Read the model definition and answer for the solid it produces. Units are mm, in the model's axes. A direction names the side the tool comes from. Give positions to 0.01 mm unless a question says otherwise; leave off trailing zeros. Order: outer loops, then holes, each group sorted by start corner. A loop starts at its lowest first (then second) coordinate and runs counter-clockwise, first axis right, second up. Notation, with made-up numbers: (16.25, -10.5) - (26.25, -10.5) arc R20 cw to (26.25, 1.5) - close; hole circle Ø6 at (7.25, 62.25). An arc over 180 degrees is marked (long way). Return JSON: item names as keys, results as strings.
```python
from build123d import *

# Parameters (mm, degrees)
SKETCH_3_R          = 1.25
CUT_EXTRUDE_1_DEPTH = 15.361406616
CHAMFER_1_SIZE      = 0.2


with BuildPart() as part:
    # 草图2 → 旋转1 (revolve)
    with BuildSketch(Plane.XY, mode=Mode.PRIVATE) as revolve_1_sk:
        Polygon((0, 3), (0, 4.5), (2, 4.5), (2, 10), (4.5, 10), (4.5, 1.5), (3.5, 1.5), (3.5, 3), align=None)
    revolve(revolve_1_sk.sketch.rotate(Axis((0, 0, 0), (1, 0, 0)), 90), axis=Axis((0, 0, 0), (1, 0, 0)))

    # 草图3 → 切除-拉伸1 (cut, through all)
    with BuildSketch(Plane.ZY.offset(-2)):
        with Locations((4.949747468, 4.949747468)):
            Circle(SKETCH_3_R)
        with Locations((4.949747468, -4.949747468)):
            Circle(SKETCH_3_R)
        with Locations((-4.949747468, -4.949747468)):
            Circle(SKETCH_3_R)
        with Locations((-4.949747468, 4.949747468)):
            Circle(SKETCH_3_R)
    extrude(amount=-CUT_EXTRUDE_1_DEPTH, mode=Mode.SUBTRACT)

    # 倒角1
    chamfer_1_edges = [part.edges().sort_by_distance(p)[0] for p in [
        (4.5, 0, -1.5),
        (4.5, 0, -10),
        (2, 0, -10),
        (0, 0, -4.5),
    ]]
    chamfer(chamfer_1_edges, length=CHAMFER_1_SIZE)


solid = part.part
```
Q1. A cutting plane is placed at C-C (x = 1). Write down the section's boundary in (y, z).
Values:
{"outline": "circle Ø9 at (0, 0); hole circle Ø6 at (0, 0)"}
Q2. For faces 4 (the cylindrical face through (1.11, -3.04, -3.32)), 5 (the flat face through (0, 1, 3)), determine the directions among +Z, -Z, +X, -X, +Y, -Y from which every point of the face is accessible in a straight line to the end or side of a thin tool.
Values:
{"face 4": "-X", "face 5": "+Z, -Z, -X, +Y, -Y"}
Q3. A cutting plane is placed at D-D (y = 4). Give the number of separate pieces and of enclosed holes in the cut face, and give its area (3 significant figures).
Values:
{"separate pieces": "3", "enclosed holes": "0", "area": "45.8 mm²"}
Q4. Consider L1, parallel to X at y = 2.25, z = 1; L2, parallel to Z at x = 1.9, y = 1.5; L3, parallel to Y at x = 3.1, z = 5.5. Determine where each line is inside the solid, lowest interval first.
Values:
{"L1": "x = 3.5 to 4.5", "L2": "z = -4.24 to -2.6, 2.6 to 4.24", "L3": "y = -8.35 to -6.07, -3.83 to 3.83, 6.07 to 8.35"}
Q5. Determine the mould class of faces 1 (the flat face through (4.5, 0, 2)), 2 (the cylindrical face through (3.23, -6.17, 4.68)), 3 (the cylindrical face through (3, 0, -10)) for opening direction Y: released by +Y, released by -Y, zero draft, split by the parting line, or undercut.
Values:
{"face 1": "zero draft", "face 2": "undercut", "face 3": "split by the parting line"}
Q6. Given pin 1 (6 mm diameter, centred on y = -1, z = -3.5, fed in from -X); pin 2 (2 mm diameter, centred on x = 1.5, y = -3.5, fed in from +Z); pin 3 (3 mm diameter, centred on y = -1, z = 1, fed in from -X); pin 4 (1.5 mm diameter, centred on y = -7.5, z = 1.5, fed in from -X), each flat-ended and moving along its own axis, determine where each tip first touches the part or whether it passes through.
Values:
{"pin 1": "stops at x = 0", "pin 2": "stops at z = 9.6", "pin 3": "stops at x = 3.5", "pin 4": "stops at x = 2"}
Q7. A cutting plane is placed at A-A (z = 0). Write down the section's boundary in (x, y).
Values:
{"outline": "(0, -4.3) - (0.2, -4.5) - (2, -4.5) - (2, -9.8) - (2.2, -10) - (4.3, -10) - (4.5, -9.8) - (4.5, -1.7) - (4.3, -1.5) - (3.5, -1.5) - (3.5, -3) - (0, -3) - close; (0, 3) - (3.5, 3) - (3.5, 1.5) - (4.3, 1.5) - (4.5, 1.7) - (4.5, 9.8) - (4.3, 10) - (2.2, 10) - (2, 9.8) - (2, 4.5) - (0.2, 4.5) - (0, 4.3) - close"}
